Part print with two shaded views. Sizes in mm from the minimum x, y, z corner. A direction names the side the tool comes from. Coordinates: 2 decimals unless noted, no trailing zeros. Write each loop counter-clockwise with the first axis right and the second up, starting at its lowest first coordinate (ties: lowest second). Pieces come first, ordered by that corner, then holes. Notation, with made-up numbers: (74, -0.75) - (94, -0.75) arc R14 ccw to (94, 9.25) - close; hole circle Ø7 at (38.25, 52.5). An arc over 180 degrees is marked (long way). Answer in a Markdown table with one row per item. Add a question column.
Q1. Drill centre lines: line 1 along Z through (x, y) = (1.2, 1.9); line 2 along Z through (x, y) = (4.5, 1.3); line 3 along X through (y, z) = (4.1, 20.5). Where is each one in solid material? Low to high. Write a range as from..to.
Q2. Band-saw the part on C-C (z = 20.25). List the corners of the cut face in (x, y), and give its area (3 significant figures).
Q3. Band-saw the part on D-D (z = 10.5). List the corners of the cut face in (x, y).
Q4. Band-saw the part on A-A (x = 2.75). List the corners of the cut face in (y, z).
Q5. 3-axis set-ups, long thin cutter, end or side, ignore diameter. For the marked faces 1 and 2: which of +Z, -Z, +X, -X, +Y, -Y reach the whole face in a straight line?
Q6. Pin check, flat tips, straight feed: pin 1 (1 mm diameter, centred on x = 2, y = 3, fed in from -Z); pin 2 (2 mm diameter, centred on y = 3, z = 11, fed in from -X); pin 3 (2 mm diameter, centred on x = 2.5, z = 15, fed in from +Y); pin 4 (1 mm diameter, centred on y = 2, z = 12.5, fed in from +X). Stop position of each tip, or through.
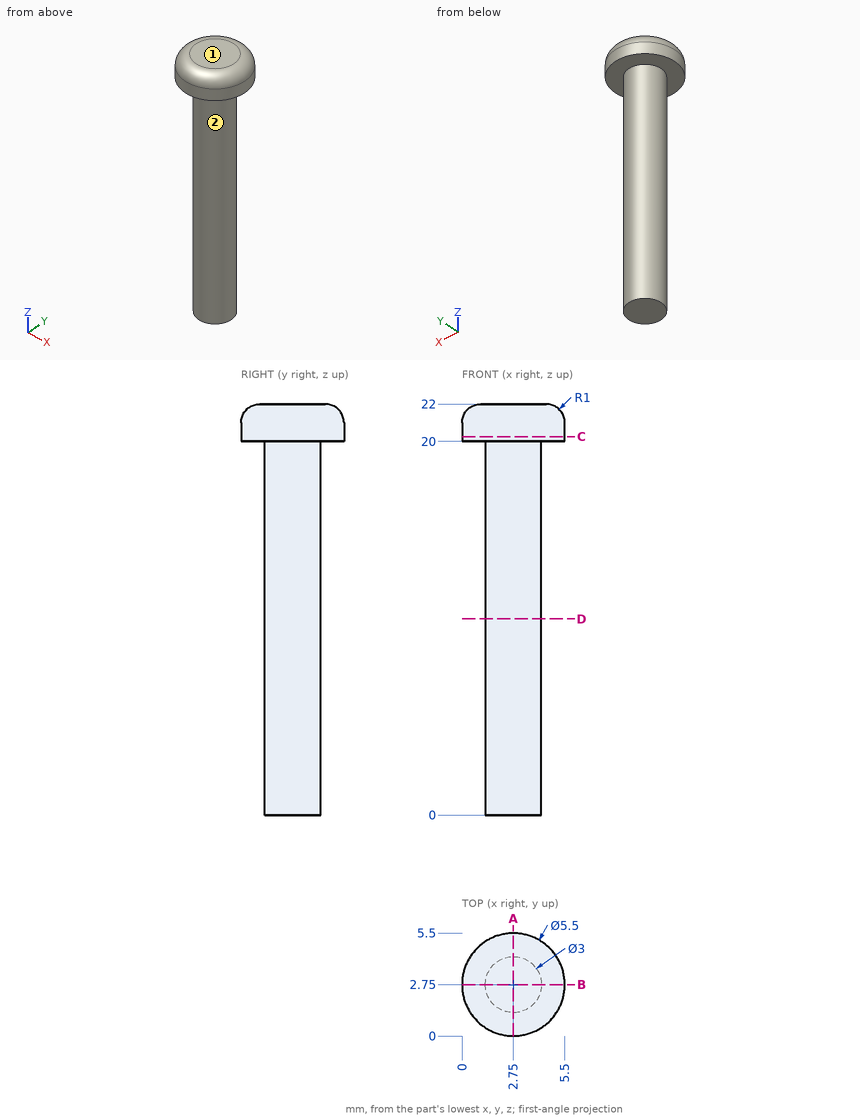
Checked values:
| question | item | result |
|---|---|---|
| 1 | line 1 | z = 20..22 |
| 1 | line 2 | z = 20..21.85 |
| 1 | line 3 | x = 0.35..5.15 |
| 2 | outline | circle Ø5.5 at (2.75, 2.75) |
| 2 | area | 23.8 mm² |
| 3 | outline | circle Ø3 at (2.75, 2.75) |
| 4 | outline | (0, 20) - (1.25, 20) - (1.25, 0) - (4.25, 0) - (4.25, 20) - (5.5, 20) - (5.5, 21) arc R1 ccw to (4.5, 22) - (1, 22) arc R1 ccw to (0, 21) - close |
| 5 | face 1 | +Z, +X, -X, +Y, -Y |
| 5 | face 2 | -Z |
| 6 | pin 1 | stops at z = 0 |
| 6 | pin 2 | stops at x = 1.25 |
| 6 | pin 3 | stops at y = 4.25 |
| 6 | pin 4 | stops at x = 4.23 |
